```python
from build123d import *

# Parameters (mm, degrees)
BOSS_EXTRU_1_DEPTH      = 6.35
ENL_V_MAT_EXTRU_2_DEPTH = 198.361432403
CONG_1_R                = 6.35


with BuildPart() as part:
    # Esquisse2 → Boss.-Extru.1 (new body)
    with BuildSketch(Plane.XY):
        Polygon((6.35, -190.5), (12.7, -190.5), (12.7, 190.5), (-12.7, 190.5), (-12.7, -190.5), (-6.35, -190.5), (-6.35, -196.85), (6.35, -196.85), align=None)
    extrude(amount=BOSS_EXTRU_1_DEPTH)

    # Esquisse4 → Enlèv. mat.-Extru.2 (cut, through all)
    with BuildSketch(Plane.XY.offset(6.35)):
        with BuildLine():
            Line((2.75, 165.1), (2.75, 38.1))
            ThreePointArc((2.75, 38.1), (0, 35.35), (-2.75, 38.1))
            Line((-2.75, 38.1), (-2.75, 165.1))
            ThreePointArc((-2.75, 165.1), (0, 167.85), (2.75, 165.1))
        make_face()
    extrude(amount=-ENL_V_MAT_EXTRU_2_DEPTH, mode=Mode.SUBTRACT)

    # Congé1
    cong_1_edges = [part.edges().sort_by_distance(p)[0] for p in [
        (-12.7, 190.5, 3.175),
        (12.7, 190.5, 3.175),
    ]]
    fillet(cong_1_edges, radius=CONG_1_R)


solid = part.part
```
Can you work these out from the model? Positions are in its coordinate system, mm. A direction names the side the tool comes from. Give positions to 0.01 mm unless a question says otherwise; leave off trailing zeros. Write each loop counter-clockwise with the first axis right and the second up, starting at its lowest first coordinate (ties: lowest second). Pieces come first, ordered by that corner, then holes. Notation, with made-up numbers: (-37.5, 88) - (-10.5, 88) arc R22 ccw to (-10.5, 115) - close; hole circle Ø6 at (-34.75, -1). An arc over 180 degrees is marked (long way). Write item = value, one per line. Start each with the question number.
1. Thinking about a two-plate mould opening in Y: for faces 5 (the face through (0, 0, 6.35)), 6 (the face through (-10, -190.5, 3)), 7 (the face through (-2.75, 101, 3)), which applies, released by +Y, released by -Y, zero draft, split by the parting line, or undercut?
2. Imagine slicing it at B-B (z = 2.5). Please give me the cut outline in (x, y), and give its area (3 significant figures).
3. On a 3-axis mill with a long thin cutter (end or side, diameter ignored), from which of +Z, -Z, +X, -X, +Y, -Y can I reach the whole of each face in a straight line? I mean faces 1 (the face through (-6.35, -194, 3)), 2 (the face through (6.35, -194, 3)), 3 (the face through (12.7, -6, 3)), 4 (the face through (2.75, 102, 3)). Say none if no direction works.
4. Imagine slicing it at A-A (y = 134). Please give me the cut outline in (x, z), and give its area (3 significant figures).
5. For pin 1 (1.9 mm diameter, centred on y = -194.5, z = 4, fed in from +X), with a flat end and sliding along its axis, tell me the tip position at first contact or that it passes through.
6. Please list where these lines run through material, in increasing order: line 1 (X direction, y = 163, z = 4); line 2 (Y direction, x = -0.5, z = 4.75); line 3 (Y direction, x = 7, z = 5).
Worked answers:
q1.face_5 = zero draft
q1.face_6 = released by -Y
q1.face_7 = undercut
q2.outline = (-12.7, -190.5) - (-6.35, -190.5) - (-6.35, -196.85) - (6.35, -196.85) - (6.35, -190.5) - (12.7, -190.5) - (12.7, 184.15) arc R6.35 ccw to (6.35, 190.5) - (-6.35, 190.5) arc R6.35 ccw to (-12.7, 184.15) - close; hole (-2.75, 38.1) arc R2.75 ccw to (2.75, 38.1) - (2.75, 165.1) arc R2.75 ccw to (-2.75, 165.1) - close
q2.area = 9,020 mm2
q3.face_1 = +Z, -Z, -X, -Y
q3.face_2 = +Z, -Z, +X, -Y
q3.face_3 = +Z, -Z, +X, +Y, -Y
q3.face_4 = +Z, -Z
q4.outline = (-12.7, 0) - (-2.75, 0) - (-2.75, 6.35) - (-12.7, 6.35) - close; (2.75, 0) - (12.7, 0) - (12.7, 6.35) - (2.75, 6.35) - close
q4.area = 126 mm2
q5.pin_1 = 6.35
q6.line_1 = -12.7 to -2.75, 2.75 to 12.7
q6.line_2 = -196.85 to 35.4, 167.8 to 190.5
q6.line_3 = -190.5 to 190.47
